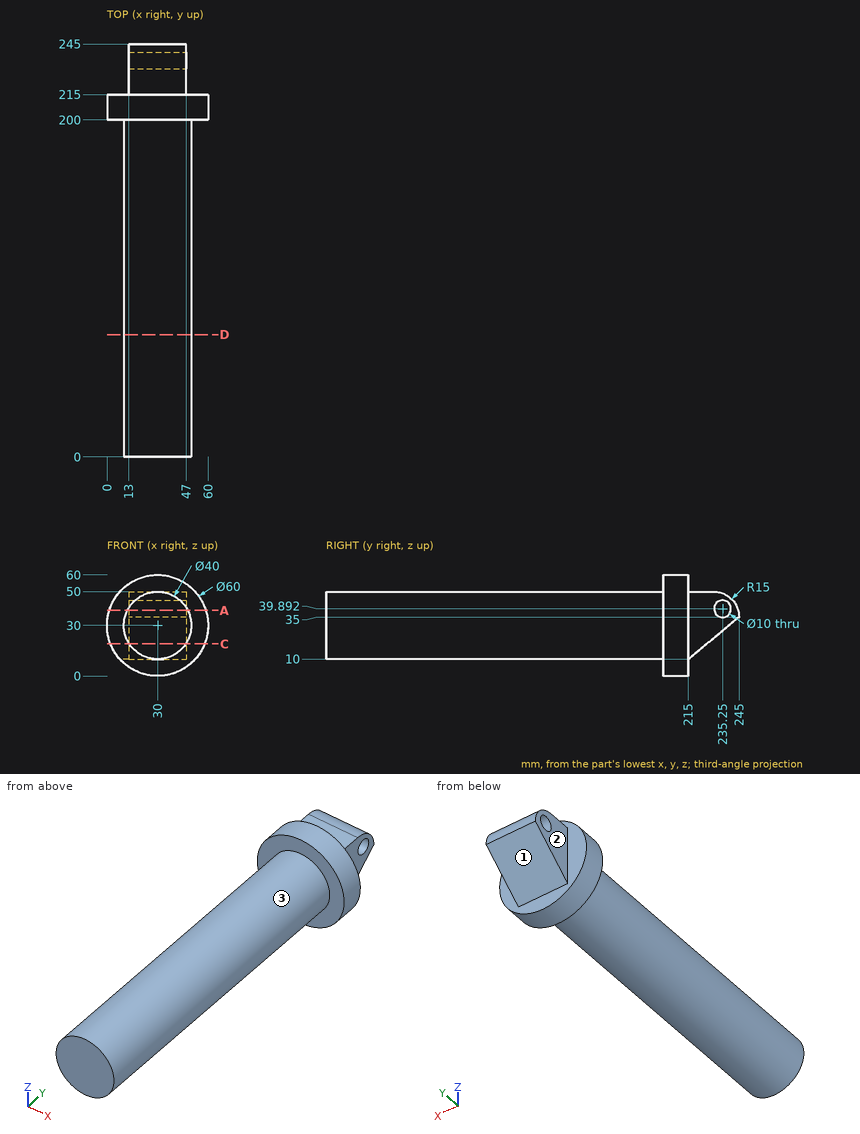
Input: dimensioned drawing with shaded views. Units: mm. Origin: part minimum x, y, z. A direction names the side the tool comes from. Give positions to 0.01 mm unless a question says otherwise; leave off trailing zeros. Write each loop counter-clockwise with the first axis right and the second up, starting at its lowest first coordinate (ties: lowest second). Pieces come first, ordered by that corner, then holes. Notation, with made-up numbers: M -27,56 L -20,56 A23 ccw -20,78 Z; hole C 1,41 d8. An arc over 180 degrees is marked long. Write item = value, one per line. Start each with the question number.
1) Cut plane A-A on z = 39. Return the cut outline in (x, y).
2) Reachability of the marked faces 1, 2 and 3 from +Z, -Z, +X, -X, +Y, -Y: full face, straight path, thin tool, end or side. Return the list, or none.
3) Cut plane D-D on y = 72.5. Return the cut outline in (x, z).
4) Material intervals for line 1 along Z through (x, y) = (29.5, 86.5); line 2 along Y through (x, z) = (19, 36.5) (1 decimal); line 3 along Y through (x, z) = (42.5, 3), sorted ascending. Write a range as [from, to].
5) First-contact query: pin 1 Ø1 at (x, y) = (44.5, 212.5) entering from +Z; pin 2 Ø6 at (y, z) = (40.5, 41.5) entering from +X; pin 3 Ø5 at (x, y) = (38.5, 191.5) entering from -Z; pin 4 Ø5 at (x, y) = (54, 46) entering from -Z. Flat tips, straight axial feed; report the tip coordinate or a pass-through.
6) Cut plane C-C on z = 19. Return the cut outline in (x, y).
Solved:
q1.outline = M 1.38,200 L 12.14,200 L 12.14,0 L 47.86,0 L 47.86,200 L 58.62,200 L 58.62,215 L 47,215 L 47,230.33 L 13,230.33 L 13,215 L 1.38,215 Z; M 13,240.17 L 47,240.17 L 47,244.46 L 13,244.46 Z
q2.face_1 = -Z, +X, -X, +Y
q2.face_2 = +Z, -Z, -X, +Y
q2.face_3 = -Y
q3.outline = C 30,30 d40
q4.line_1 = [10.01, 49.99]
q4.line_2 = [0, 231.6], [238.9, 244.9]
q4.line_3 = [200, 215]
q5.pin_1 = 56.53
q5.pin_2 = 48.1
q5.pin_3 = 10.92
q5.pin_4 = through
q6.outline = M 2.09,200 L 13.3,200 L 13.3,0 L 46.7,0 L 46.7,200 L 57.91,200 L 57.91,215 L 47,215 L 47,225.8 L 13,225.8 L 13,215 L 2.09,215 Z
